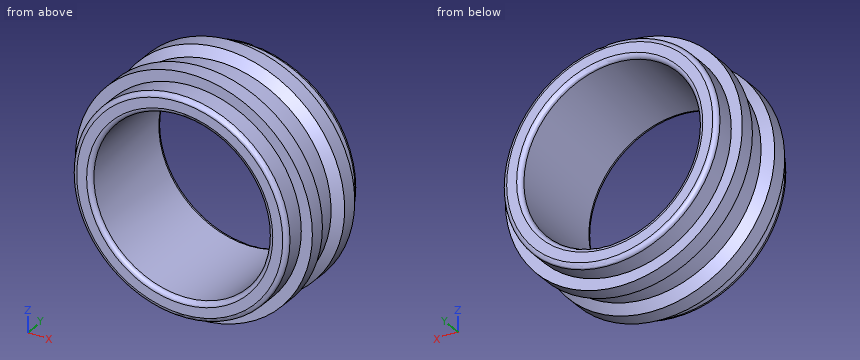
from build123d import *

# Parameters (mm, degrees)
IZIM1_R                     = 5.35
IZIM1_R_2                   = 4
Y_KSEKLIK_EKSTR_ZYON1_DEPTH = 5
IZIM4_R                     = 5.35
IZIM4_R_2                   = 4.85
KES_EKSTR_ZYON1_DEPTH       = 1
L_O_ALTMA1_COUNT            = 2
L_O_ALTMA1_PITCH            = 4
RADYUS1_R                   = 0.2


with BuildPart() as part:
    # Çizim1 → Yükseklik-Ekstrüzyon1 (new body)
    with BuildSketch(Plane(origin=(0, 0, 0), x_dir=(1, 0, 0), z_dir=(0, 1, 0))):
        Circle(IZIM1_R)
        Circle(IZIM1_R_2, mode=Mode.SUBTRACT)
    extrude(amount=Y_KSEKLIK_EKSTR_ZYON1_DEPTH)

    # Çizim4 → Kes-Ekstrüzyon1 (cut)
    with BuildSketch(Plane(origin=(0, 5, 0), x_dir=(1, 0, 0), z_dir=(0, 1, 0))):
        Circle(IZIM4_R)
        Circle(IZIM4_R_2, mode=Mode.SUBTRACT)
    kes_ekstr_zyon1 = extrude(amount=-KES_EKSTR_ZYON1_DEPTH, mode=Mode.SUBTRACT)

    # LÇoğaltma1: Kes-Ekstrüzyon1 ×2
    with Locations(*[(0, -i * L_O_ALTMA1_PITCH, 0) for i in range(1, L_O_ALTMA1_COUNT)]):
        add(kes_ekstr_zyon1, mode=Mode.SUBTRACT)

    # Çizim6 → Kes-Döndür1 (revolve, cut)
    with BuildSketch(Plane.XY):
        Polygon((-5.560786438, 3.5), (-4.975, 2.914213562), (-4.975, 2.085786438), (-5.560786438, 1.5), align=None)
    revolve(axis=Axis((0, 0, 0), (0, 1, 0)), mode=Mode.SUBTRACT)

    # Radyus1
    radyus1_edges = [part.edges().sort_by_distance(p)[0] for p in [
        (-4.85, 5, 0),
        (-4.85, 0, 0),
        (-4, 0, 0),
        (-4, 5, 0),
    ]]
    fillet(radyus1_edges, radius=RADYUS1_R)


solid = part.part
Work out the finished part from the listing and answer in its coordinate system (mm). Coordinates: 2 decimals unless noted, no trailing zeros. Loops run counter-clockwise (first coordinate to the right, second up) from the corner with the lowest first, then second, coordinate; pieces in that order, holes last. Notation, with made-up numbers: (74, -11) -> (124, -11) arc R27 cw to (124, 15) -> close; hole circle Ø6 at (14, -4). An arc over 180 degrees is marked (long way). Write each question's results on one line, items separated by ' | '. Start each with the question number.
1) Find section C-C on y = 0.4. Determine the outline of the cut face in (x, z), then the cut area to 3 significant figures.
2) Find section D-D on y = 2.55. Determine the outline of the cut face in (x, z) (3 decimals).
3) Consider line 1 along X through (y, z) = (3.75, 0); line 2 along X through (y, z) = (4.7, 0.5); line 3 along Z through (x, y) = (-2.25, 0.4). Determine where each line is inside the solid, lowest interval first.
4) A flat-ended cylindrical pin translates along its axis: P1, Ø1.5, axis at y = 3, z = -2.5, coming from the +X side. Find the tip coordinate at first contact, or state that the pin passes through.
Response values:
1) outline: circle Ø9.7 at (0, 0); hole circle Ø8 at (0, 0) | area: 23.6 mm^2
2) outline: circle Ø9.95 at (0, 0); hole circle Ø8 at (0, 0)
3) line 1: x = -5.35 to -4, 4 to 5.35 | line 2: x = -4.82 to -3.97, 3.97 to 4.82 | line 3: z = -4.3 to -3.31, 3.31 to 4.3
4) P1: stops at x = 5.04
